Design review of the part built by this model. Coordinates are the model's own, in mm. A direction names the side the tool comes from. Coordinates: 2 decimals unless noted, no trailing zeros. Order: outer loops, then holes, each group sorted by start corner. A loop starts at its lowest first (then second) coordinate and runs counter-clockwise, first axis right, second up. Notation, with made-up numbers: M 29.25,15.25 L 67.25,15.25 A6 ccw 67.25,22.25 Z; hole C 81,5 d2. An arc over 180 degrees is marked long. Answer as a JSON object with one key per item and string values.
from build123d import *

# Parameters (mm, degrees)
RESSALTO_EXTRUS_O1_DEPTH = 5
BOSS_EXTRUDE1_DEPTH      = 10
CUT_EXTRUDE1_DEPTH       = 50
SKETCH3_W                = 10
SKETCH3_H                = 3.990496563
CUT_EXTRUDE2_DEPTH       = 12


with BuildPart() as part:
    # Esboço1 → Ressalto-extrusão1 (new, symmetric)
    with BuildSketch(Plane.XY):
        Polygon((-2.596479089, -162.874745928), (2.546479089, -161.115750635), (2.546479089, -158.884249365), (-2.596479089, -157.125254072), (-2.596479089, -154.874745928), (2.546479089, -153.115750635), (2.546479089, -150.884249365), (-2.596479089, -149.125254072), (-2.596479089, -146.874745928), (2.546479089, -145.115750635), (2.546479089, -142.884249365), (-2.596479089, -141.125254072), (-2.596479089, -138.874745928), (2.546479089, -137.115750635), (2.546479089, -134.884249365), (-2.596479089, -133.125254072), (-2.596479089, -130.874745928), (2.546479089, -129.115750635), (2.546479089, -126.884249365), (-2.596479089, -125.125254072), (-2.596479089, -122.874745928), (2.546479089, -121.115750635), (2.546479089, -118.884249365), (-2.596479089, -117.125254072), (-2.596479089, -114.874745928), (2.546479089, -113.115750635), (2.546479089, -110.884249365), (-2.596479089, -109.125254072), (-2.596479089, -106.874745928), (2.546479089, -105.115750635), (2.546479089, -102.884249365), (-2.596479089, -101.125254072), (-2.596479089, -98.874745928), (2.546479089, -97.115750635), (2.546479089, -94.884249365), (-2.596479089, -93.125254072), (-2.596479089, -90.874745928), (2.546479089, -89.115750635), (2.546479089, -86.884249365), (-2.596479089, -85.125254072), (-2.596479089, -82.874745928), (2.546479089, -81.115750635), (2.546479089, -78.884249365), (-2.596479089, -77.125254072), (-2.596479089, -74.874745928), (2.546479089, -73.115750635), (2.546479089, -70.884249365), (-2.596479089, -69.125254072), (-2.596479089, -66.874745928), (2.546479089, -65.115750635), (2.546479089, -62.884249365), (-2.596479089, -61.125254072), (-2.596479089, -58.874745928), (2.546479089, -57.115750635), (2.546479089, -54.884249365), (-2.596479089, -53.125254072), (-2.596479089, -50.874745928), (2.546479089, -49.115750635), (2.546479089, -46.884249365), (-2.596479089, -45.125254072), (-2.596479089, -42.874745928), (2.546479089, -41.115750635), (2.546479089, -38.884249365), (-2.596479089, -37.125254072), (-2.596479089, -34.874745928), (2.546479089, -33.115750635), (2.546479089, -30.884249365), (-2.596479089, -29.125254072), (-2.596479089, -26.874745928), (2.546479089, -25.115750635), (2.546479089, -22.884249365), (-2.596479089, -21.125254072), (-2.596479089, -18.874745928), (2.546479089, -17.115750635), (2.546479089, -14.884249365), (-2.596479089, -13.125254072), (-2.596479089, -10.874745928), (2.546479089, -9.115750635), (2.546479089, -6.884249365), (-2.596479089, -5.125254072), (-2.596479089, -2.874745928), (2.546479089, -1.115750635), (2.546479089, 1.115750635), (-2.596479089, 2.874745928), (-2.596479089, 5.125254072), (2.546479089, 6.884249365), (2.546479089, 9.115750635), (-12.782395447, 9.115750635), (-12.782395447, -164), (-2.596479089, -164), align=None)
    extrude(amount=RESSALTO_EXTRUS_O1_DEPTH, both=True)

    # Sketch1 → Boss-Extrude1 (add)
    with BuildSketch(Plane(origin=(0, 9.115750635, 0), x_dir=(1, 0, 0), z_dir=(0, 1, 0))):
        Polygon((2.782395447, 5), (-12.782395447, 5), (-12.782395447, -5), (2.782395447, -5), (2.782395447, -11.950821596), (7.782395447, -11.950821596), (12.782395447, -11.950821596), (12.782395447, -1.100821596), (7.782395447, -1.100821596), (-5.426721346, -1.100821596), (-5.426721346, 1.100821596), (2.782395447, 1.100821596), (12.782395447, 1.100821596), (12.782395447, 11.946726984), (7.782395447, 11.946726984), (2.782395447, 11.946726984), align=None)
    extrude(amount=BOSS_EXTRUDE1_DEPTH)

    # Sketch2 → Cut-Extrude1 (cut)
    with BuildSketch(Plane(origin=(0, 19.115750635, 0), x_dir=(1, 0, 0), z_dir=(0, 1, 0))):
        Polygon((10.616582745, 13.051407562), (13.445399336, 13.051407562), (13.445399336, -14.793690682), (10.616582745, -14.793690682), (5.402017224, -14.793690682), (5.402017224, 13.051407562), align=None)
    extrude(amount=-CUT_EXTRUDE1_DEPTH, mode=Mode.SUBTRACT)

    # Sketch3 → Cut-Extrude2 (cut)
    with BuildSketch(Plane(origin=(2.546479089, 0, 0), x_dir=(0, 0, -1), z_dir=(1, 0, 0))):
        with Locations((0, 7.120502354)):
            Rectangle(SKETCH3_W, SKETCH3_H)
    extrude(amount=-CUT_EXTRUDE2_DEPTH, mode=Mode.SUBTRACT)


solid = part.part
1) Tool access review of faces 1 (the flat face through (-12.782, -74, 0)), 2 (the flat face through (-0.061, -66.008, 0.07)): name each direction out of +Z, -Z, +X, -X, +Y, -Y from which nothing blocks a thin tool from reaching the whole face with its end or side.
Taken from the geometry:
{"face 1": "+Z, -Z, -X, +Y, -Y", "face 2": "+Z, -Z, +X"}
2) To check wall thickness, follow L1, parallel to Y at x = -9, z = 0.25; L2, parallel to X at y = -48, z = 4.5; L3, parallel to Z at x = -4.5, y = 3. State the ranges of each line that lie inside material, in increasing order.
Taken from the geometry:
{"L1": "y = -164 to 5.13, 9.12 to 19.12", "L2": "x = -12.78 to 2.55", "L3": "z = -5 to 5"}
3) Insertion check: pin 1 Ø1.1 at (y, z) = (0, 0.5) entering from +X; pin 2 Ø6 at (x, z) = (3, -2) entering from -Y; pin 3 Ø1.8 at (y, z) = (-12, -1.5) entering from +X; pin 4 Ø2.5 at (y, z) = (14, -0.5) entering from +X. Each pin has a flat end and moves straight along its axis. Give the tip position at first contact, or say it passes through.
Taken from the geometry:
{"pin 1": "stops at x = 2.55", "pin 2": "stops at y = -161.99", "pin 3": "stops at x = -2.6", "pin 4": "stops at x = 5.4"}
4) Mouldability with a two-part tool opening along Y and no side actions: class faces 3 (the flat face through (-8, -164, 0)), 4 (the flat face through (-2, 19.116, -2)), 5 (the flat face through (0.011, -6.017, 0.07)) as released by +Y, released by -Y, zero draft, split by the parting line, or undercut.
Taken from the geometry:
{"face 3": "released by -Y", "face 4": "released by +Y", "face 5": "undercut"}
5) Add section A-A (x = -1). Count the separate pieces of the cut face and the enclosed holes in it, and give its area (3 significant figures).
Taken from the geometry:
{"separate pieces": "23", "enclosed holes": "0", "area": "1,060 mm2"}
6) Add section B-B (z = -8.75). State the section outline as (x, y) points.
Taken from the geometry:
{"outline": "M 2.78,9.12 L 5.4,9.12 L 5.4,19.12 L 2.78,19.12 Z"}
